Input: part model. Units: mm. Frame: model coordinates. A direction names the side the tool comes from. Give positions to 0.01 mm unless a question says otherwise; leave off trailing zeros. Write each loop counter-clockwise with the first axis right and the second up, starting at its lowest first coordinate (ties: lowest second). Pieces come first, ordered by that corner, then holes.
Autodesk Inventor part; units mm, degrees
ref_plane "YZ Plane" through (0, 0, 0) normal (1, 0, 0) x (0, 1, 0)
ref_plane "XZ Plane" through (0, 0, 0) normal (0, 1, 0) x (-1, 0, 0)
ref_plane "XY Plane" through (0, 0, 0) normal (0, 0, 1) x (1, 0, 0)
sketch "Sketch1" plane through (0, 0, 0) normal (0, 0, 1) x (1, 0, 0)
  circle A0 centre (-20.2579, 7.5645) radius 2.5
  line L0 (34.7421, -2.4355) -> (34.7421, 2.5645)
  line L1 (34.7421, 2.5645) -> (-15.2579, 2.5645)
  line L2 (-15.2579, 2.5645) -> (-15.2579, 7.5645)
  arc A1 (-15.2579, 7.5645) -> (-25.2579, 7.5645) centre (-20.2579, 7.5645) ccw
  line L3 (-25.2579, 7.5645) -> (-25.2579, -62.4355)
  line L4 (-25.2579, -62.4355) -> (4.7421, -62.4355)
  line L5 (9.7421, -57.4355) -> (4.7421, -62.4355)
  line L6 (-20.2579, -57.4355) -> (9.7421, -57.4355)
  line L7 (-20.2579, -2.4355) -> (-20.2579, -57.4355)
  line L8 (-20.2579, -2.4355) -> (34.7421, -2.4355)
  line L9 (-15.2579, 2.5645) -> (-25.2579, 2.5645)
  point P0 (0, 0)
  point P1 (4.7421, 37.5645)
  dimension "d0" = 5
  dimension "d1" = 5
  dimension "d2" = 30
  dimension "d3" = 55
  dimension "d4" = 5
  dimension "d5" = 5
  dimension "d6" = 5
  dimension "d7" = 65
  dimension "d8" = 5
  dimension "d24" = 30
extrude "Extrusion1" add sketch "Sketch1" along normal blind 25
ref_plane "Work Plane1" through (0, 0, 12.5) normal (0, 0, 1) x (1, 0, 0)
sketch "Sketch2" plane through (0, 0, 12.5) normal (0, 0, 1) x (1, 0, 0)
  line L0 (-15.2579, 2.5645) -> (-15.2579, 7.5645)
  line L1 (34.7421, 2.5645) -> (-15.2579, 2.5645)
  line L2 (34.7421, -2.4355) -> (34.7421, 2.5645)
  line L3 (-20.2579, -2.4355) -> (34.7421, -2.4355)
  line L4 (-20.2579, -57.4355) -> (-20.2579, -2.4355)
  line L5 (9.7421, -57.4355) -> (-20.2579, -57.4355)
  line L6 (4.7421, -62.4355) -> (9.7421, -57.4355)
  line L7 (-25.2579, -62.4355) -> (4.7421, -62.4355)
  line L8 (-25.2579, 7.5645) -> (-25.2579, -62.4355)
  arc A0 (-15.2579, 7.5645) -> (-25.2579, 7.5645) centre (-20.2579, 7.5645) ccw
  circle A1 centre (-20.2579, 7.5645) radius 2.5
  line L9 (-15.2579, 2.5645) -> (-15.2579, 7.5645)
  line L10 (-15.2579, 2.5645) -> (-25.2579, 2.5645)
  line L11 (-25.2579, 7.5645) -> (-25.2579, -62.4355)
  point P0 (0, 0)
extrude "Extrusion2" cut sketch "Sketch2" along normal mid plane 19 contours L10 L8 A0 L0
sketch "Sketch3" plane through (0, 0, 12.5) normal (0, 0, 1) x (1, 0, 0)
  line L0 (-20.2579, -2.4355) -> (34.7421, -2.4355)
  line L1 (34.7421, -2.4355) -> (42.2421, 10.5548)
  line L2 (34.7421, -2.4355) -> (34.7421, 2.5645)
  line L3 (34.7421, 2.5645) -> (40.0771, 11.8048)
  circle A0 centre (38.8271, 9.6398) radius 1.5
  line L4 (34.7421, 2.5645) -> (-15.2579, 2.5645)
  line L5 (42.2421, 10.5548) -> (40.0771, 11.8048)
  line L6 (40.0771, 11.8048) -> (37.912, 13.0548)
  line L7 (37.912, 13.0548) -> (31.8554, 2.5645)
  circle A1 centre (38.8271, 9.6398) radius 2.5
  point P0 (0, 0)
  point P1 (36.662, 10.8898)
  point P2 (40.9921, 8.3898)
  dimension "d13" = 15
  dimension "d14" = 30
  dimension "d15" = 3
  dimension "d16" = 2.5
  dimension "d17" = 60
  dimension "d18" = 2.5
  dimension "d19" = 2.5
extrude "Extrusion3" add sketch "Sketch3" along normal mid plane 25 contours L2 L3 A1 L1 | A1 L3 A0 | L4 L7 A1 L3 | A1 L3 A0
extrude "Extrusion4" cut sketch "Sketch3" along normal mid plane 19 contours L2 L3 A1 L1 | A1 L3 A0 | L4 L7 A1 L3 | A1 L3 A0
sketch "Sketch4" plane through (0, 0, 0) normal (0, 0, -1) x (-1, 0, 0)
  circle A0 centre (-38.8271, 9.6398) radius 1.5
  line L0 (15.2579, 2.5645) -> (15.2579, 7.5645)
  line L1 (-31.8554, 2.5645) -> (15.2579, 2.5645)
  line L2 (-31.8554, 2.5645) -> (-36.662, 10.8898)
  arc A1 (-36.662, 10.8898) -> (-40.9921, 8.3898) centre (-38.8271, 9.6398) ccw
  line L3 (-40.9921, 8.3898) -> (-34.7421, -2.4355)
  line L4 (20.2579, -2.4355) -> (-34.7421, -2.4355)
  line L5 (20.2579, -57.4355) -> (20.2579, -2.4355)
  line L6 (-9.7421, -57.4355) -> (20.2579, -57.4355)
  line L7 (-4.7421, -62.4355) -> (-9.7421, -57.4355)
  line L8 (25.2579, -62.4355) -> (-4.7421, -62.4355)
  line L9 (25.2579, 7.5645) -> (25.2579, -62.4355)
  arc A2 (25.2579, 7.5645) -> (15.2579, 7.5645) centre (20.2579, 7.5645) ccw
  circle A3 centre (20.2579, 7.5645) radius 2.5
  line L10 (20.2579, -2.4355) -> (-34.7421, -2.4355)
  line L11 (-31.8554, 2.5645) -> (-34.7421, 2.5645)
  line L12 (-34.7421, -2.4355) -> (-34.7421, 2.5645)
  line L13 (-34.7421, 2.5645) -> (-31.8554, 2.5645)
  line L14 (-31.8554, 2.5645) -> (25.2579, 2.5645)
  line L15 (25.2579, 7.5645) -> (25.2579, -62.4355)
  point P0 (0, 0)
properties part number "Claw New"
Item 1: Section B-B (z = 10.75). Return loops of the section in (x, y), and give its area (4 significant figures).
Item 2: Section C-C (x = 12.5). Return loops of the section in (y, z).
Item 3: Mould query, pull axis Z, two halves, no side actions, for faces 1 (the flat face through (37, 7, 22)), 2 (the flat face through (-20.258, -30, 12)), 3 (the flat face through (34.742, 0, 13)), 4 (the flat face through (-22, -22, 0)). Classes: +Z half, -Z half, draft (parallel to the pull), parting line (faces both ways), or undercut.
Item 4: Pin query (flat end, axial travel): pin 1 (2.5 mm diameter, centred on x = 38.83, y = 9.64, fed in from -Z); pin 2 (3.5 mm diameter, centred on y = 4, z = 23, fed in from +X); pin 3 (2 mm diameter, centred on x = 25.5, z = 17, fed in from -Y); pin 4 (1.5 mm diameter, centred on y = 0, z = 12.5, fed in from +X). Return the tip coordinate at first contact, or that it passes through.
Item 5: Section A-A (x = -10). Return loops of the section in (y, z), and give its area (3 significant figures).
Item 6: Section D-D (y = -18). Return loops of the section in (x, z).
Item 7: Ray query, line 1 (Y direction, x = -0.5, z = 5.75); line 2 (Z direction, x = 36, y = 2); line 3 (Y direction, x = 24.5, z = 6.25). Return the intervals inside material, ascending.
Item 8: Set-up query: faces 5 (the flat face through (7, -2.436, 12)), 6 (the flat face through (34.3, 6.8, 23.5)), 7 (the flat face through (37.823, 2.901, 23.521)). Return all of +Z, -Z, +X, -X, +Y, -Y with unobstructed straight access to the full face (end or side cutting, diameter ignored); none if empty.
Solved:
1. outline: (-25.26, -62.44) - (4.74, -62.44) - (9.74, -57.44) - (-20.26, -57.44) - (-20.26, -2.44) - (34.74, -2.44) - (34.74, 2.56) - (-25.26, 2.56) - close
1. area: 737.5 mm2
2. outline: (-2.44, 0) - (2.56, 0) - (2.56, 25) - (-2.44, 25) - close
3. face 1: undercut
3. face 2: draft
3. face 3: undercut
3. face 4: -Z half
4. pin 1: passes through
4. pin 2: stops at x = 39.47
4. pin 3: stops at y = -2.44
4. pin 4: stops at x = 34.74
5. outline: (-62.44, 0) - (-57.44, 0) - (-57.44, 25) - (-62.44, 25) - close; (-2.44, 0) - (2.56, 0) - (2.56, 25) - (-2.44, 25) - close
5. area: 250 mm2
6. outline: (-25.26, 0) - (-20.26, 0) - (-20.26, 25) - (-25.26, 25) - close
7. line 1: y = -62.44 to -57.44, -2.44 to 2.56
7. line 2: z = 0 to 3, 22 to 25
7. line 3: y = -2.44 to 2.56
8. face 5: +Z, -Z, +X
8. face 6: +Z, -Z, +Y
8. face 7: +Z, -Z, +X, -Y
